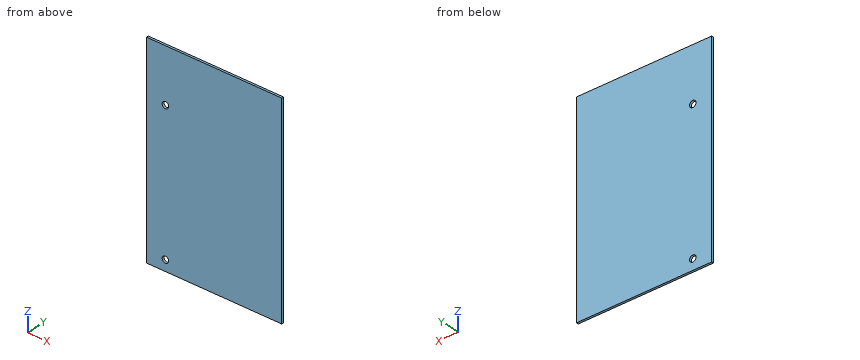
from build123d import *

# Parameters (mm, degrees)
SKETCH1_W              = 63.5
SKETCH1_H              = 96.52
BOSS_EXTRUDE1_DEPTH    = 1
SKETCH2_R              = 1.524
MOUNTING_HOLES_1_DEPTH = 2
SKETCH3_R              = 1.524
MOUNTING_HOLES_2_DEPTH = 3


with BuildPart() as part:
    # Sketch1 → Boss-Extrude1 (new body)
    with BuildSketch(Plane(origin=(0, 0, 0), x_dir=(1, 0, 0), z_dir=(0, 1, 0))):
        with Locations((31.75, 48.26)):
            Rectangle(SKETCH1_W, SKETCH1_H)
    extrude(amount=BOSS_EXTRUDE1_DEPTH)

    # Sketch2 → mounting holes (1) (cut)
    with BuildSketch(Plane(origin=(0, 1, 0), x_dir=(1, 0, 0), z_dir=(0, 1, 0))):
        with Locations(Location((8.89, 91.44, 0), (0, 0, 270))):
            Circle(SKETCH2_R)
    extrude(amount=-MOUNTING_HOLES_1_DEPTH, mode=Mode.SUBTRACT)

    # Sketch3 → mounting holes (2) (cut)
    with BuildSketch(Plane(origin=(0, 1, 0), x_dir=(1, 0, 0), z_dir=(0, 1, 0))):
        with Locations(Location((8.89, 25.4, 0), (0, 0, 270))):
            Circle(SKETCH3_R)
    extrude(amount=-MOUNTING_HOLES_2_DEPTH, mode=Mode.SUBTRACT)


solid = part.part
Design review of the part built by this model. Coordinates are the model's own, in mm. Round coordinates to 2 decimals unless told otherwise and drop trailing zeros. Write each loop counter-clockwise with the first axis right and the second up, starting at its lowest first coordinate (ties: lowest second). Pieces come first, ordered by that corner, then holes. Notation, with made-up numbers: (13.5, 16) - (28.5, 16) arc R25 ccw to (28.5, 44) - close; hole circle Ø1 at (69.25, 59.25). An arc over 180 degrees is marked (long way). Use a Markdown table: item, result. Add a question column.
1. We need section A-A (z = -25.4). State the section outline as (x, y) points.
2. Wall thickness on probe 1 along X at (y, z) = (0.7, -91.44); probe 2 along X at (y, z) = (0.8, -92): over which ranges is each line inside the solid? List them lowest first.
3. We need section B-B (x = 8.89). State the section outline as (y, z) points, then the cut area to 3 significant figures.
Output:
| question | item | result |
|---|---|---|
| 1 | outline | (0, 0) - (7.37, 0) - (7.37, 1) - (0, 1) - close; (10.41, 0) - (63.5, 0) - (63.5, 1) - (10.41, 1) - close |
| 2 | probe 1 | x = 0 to 7.37, 10.41 to 63.5 |
| 2 | probe 2 | x = 0 to 7.47, 10.31 to 63.5 |
| 3 | outline | (0, -96.52) - (1, -96.52) - (1, -92.96) - (0, -92.96) - close; (0, -89.92) - (1, -89.92) - (1, -26.92) - (0, -26.92) - close; (0, -23.88) - (1, -23.88) - (1, 0) - (0, 0) - close |
| 3 | area | 90.4 mm2 |
